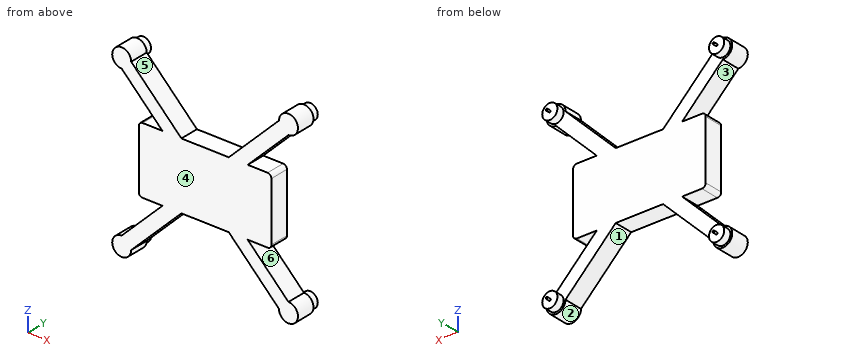
Autodesk Inventor part; units mm, degrees
ref_plane "YZ Plane" through (0, 0, 0) normal (1, 0, 0) x (0, 1, 0)
ref_plane "XZ Plane" through (0, 0, 0) normal (0, 1, 0) x (-1, 0, 0)
ref_plane "XY Plane" through (0, 0, 0) normal (0, 0, 1) x (1, 0, 0)
sketch "Sketch1" plane through (0, 0, 0) normal (0, 1, 0) x (-1, 0, 0)
  line L0 (49, 49) -> (-49, 49)
  line L1 (-49, 49) -> (-49, -49)
  line L2 (-49, -49) -> (49, -49)
  line L3 (49, -49) -> (49, 49)
  line L4 (49, 49) -> (-49, -49)
  line L5 (49, -49) -> (-49, 49)
  circle A0 centre (44, 44) radius 5
  line L6 (0, 0) -> (0, 5)
  line L7 (0, 0) -> (5, 0)
  line L8 (5, 0) -> (44, 39)
  line L9 (39, 44) -> (0, 5)
  circle A1 centre (-44, 44) radius 5
  line L10 (-44, 39) -> (-5, 0)
  line L11 (0, 5) -> (-39, 44)
  circle A2 centre (-44, -44) radius 5
  line L12 (-39, -44) -> (0, -5)
  line L13 (-5, 0) -> (-44, -39)
  circle A3 centre (44, -44) radius 5
  line L14 (44, -39) -> (5, 0)
  line L15 (0, -5) -> (39, -44)
  line L16 (-33, 17.5) -> (33, 17.5)
  line L17 (35, 15.5) -> (35, -15.5)
  line L18 (33, -17.5) -> (-33, -17.5)
  line L19 (-35, -15.5) -> (-35, 15.5)
  line L20 (-35, 17.5) -> (35, -17.5) construction
  line L21 (35, 17.5) -> (-35, -17.5) construction
  arc A4 (35, 15.5) -> (33, 17.5) centre (33, 15.5) ccw
  arc A5 (33, -17.5) -> (35, -15.5) centre (33, -15.5) ccw
  arc A6 (-35, -15.5) -> (-33, -17.5) centre (-33, -15.5) ccw
  arc A7 (-33, 17.5) -> (-35, 15.5) centre (-33, 15.5) ccw
  point P0 (12.5, 17.5)
  point P1 (-12.5, 17.5)
  point P2 (-22.5, 17.5)
  point P3 (-22.5, -17.5)
  point P4 (-12.5, -17.5)
  point P5 (12.5, -17.5)
  point P6 (22.5, -17.5)
  point P7 (22.5, 17.5)
  dimension "d0" = 98
  dimension "d1" = 98
  dimension "d2" = 10
  dimension "d3" = 49
  dimension "d4" = 49
  dimension "d7" = 360
  dimension "d10" = 70
  dimension "d11" = 35
  dimension "d12" = 2
  dimension "d13" = 2
  dimension "d14" = 2
  dimension "d15" = 2
extrude "Extrusion1" add sketch "Sketch1" along normal blind 10 contours A0 L4 | A0 L4 | A1 L5 | A0 L4 L16 L9 | A3 L5 | L8 L16 L4 A0 | L11 L16 L5 A1 | L5 A1 | L16 L4 L6 L9 | L9 L11 L16 | A3 L5 L18 L14 | A3 L5 | L16 A4 L17 A5 L18 L14 L8 | L8 L7 L4 L16 | L5 L16 L10 A1 | L11 L6 L5 L16 | A3 L15 L18 L5 | L18 L5 L7 L14 | L5 L18 L15 L12 L4 | L4 L18 L13 L10 L16 L5 | A2 L4 | A2 L4 | L18 L12 A2 L4 | L4 A2 L13 L18 | L10 L13 L18 A6 L19 A7 L16 | L18 L12 L15
sketch "Sketch2" plane through (0, 10, 0) normal (0, 1, 0) x (1, 0, 0)
  arc A0 (-44, -39) -> (-39, -44) centre (-44, -44) ccw
  circle A1 centre (-44, -44) radius 4
  arc A2 (-39, 44) -> (-44, 39) centre (-44, 44) ccw
  circle A3 centre (-44, 44) radius 4
  arc A4 (44, 39) -> (39, 44) centre (44, 44) ccw
  circle A5 centre (44, 44) radius 4
  arc A6 (39, -44) -> (44, -39) centre (44, -44) ccw
  circle A7 centre (44, -44) radius 4
  point P0 (0, 0)
  dimension "d18" = 8
  dimension "d19" = 8
  dimension "d20" = 8
  dimension "d21" = 8
extrude "Extrusion2" add sketch "Sketch2" along normal blind 4
sketch "Sketch3" plane through (-44, 14, 44) normal (0, 1, 0) x (1, 0, 0)
  circle A0 centre (0, 0) radius 0.5
  point P0 (44, 44)
  dimension "d24" = 1
sketch "Sketch4" plane through (-44, 14, -44) normal (0, 1, 0) x (1, 0, 0)
  circle A0 centre (0, 0) radius 4
  circle A1 centre (0, 0) radius 0.5
  point P0 (44, -44)
  dimension "d25" = 1
sketch "Sketch5" plane through (44, 14, -44) normal (0, 1, 0) x (1, 0, 0)
  circle A0 centre (0, 0) radius 4
  circle A1 centre (0, 0) radius 0.5
  point P0 (-44, -44)
  dimension "d26" = 1
sketch "Sketch6" plane through (44, 14, 44) normal (0, 1, 0) x (1, 0, 0)
  circle A0 centre (0, 0) radius 4
  circle A1 centre (0, 0) radius 0.5
  point P0 (-44, 44)
  dimension "d27" = 1
extrude "Extrusion3" add sketch "Sketch6" along normal blind 2 contours A1
extrude "Extrusion4" add sketch "Sketch3" along normal blind 2
extrude "Extrusion5" add sketch "Sketch4" along normal blind 2 contours A1
extrude "Extrusion6" add sketch "Sketch5" along normal blind 2 contours A1
properties part number "DroneBase"
Build history of the part. All positions in model axes, mm. Face numbers are marked on the shaded views. A direction names the side the tool comes from. Coordinates: 2 decimals unless noted, no trailing zeros. Order: outer loops, then holes, each group sorted by start corner. A loop starts at its lowest first (then second) coordinate and runs counter-clockwise, first axis right, second up. Notation, with made-up numbers: M 83,-36 L 102,-36 A12 ccw 102,-31 Z; hole C 17,-39 d9. An arc over 180 degrees is marked long. One line per question, with ' | ' between items. Start each with the question number.
1. Mould opens along X. For the marked faces 4, 5 and 6 say: +X half, -X half, draft (parallel to the pull), parting line (faces both ways), or undercut.
2. Cut at B-B (y = 5). Write the cut outline in (x, z), plus the area to 3 significant figures.
3. Flat gauge pins, fed straight in: P1, Ø8, axis at x = 30, y = 6, coming from the +Z side; P2, Ø3, axis at x = 5.5, y = 3, coming from the -Z side; P3, Ø5, axis at y = 3.5, z = 4.5, coming from the +X side; P4, Ø5, axis at y = 13, z = 13, coming from the +X side. Where does each tip first touch, or does it go through?
4. Cut at D-D (x = -9). Write the cut outline in (y, z), plus the area to 3 significant figures.
5. Cut at C-C (z = 9). Write the cut outline in (x, y), plus the area to 3 significant figures.
6. Wall check: line 1 along Z through (x, y) = (-25, 3); line 2 along Z through (x, y) = (31.5, 3.25); line 3 along Z through (x, y) = (44, 2). Give the ranges that are in metal, low to high. Write a range as [from, to].
7. Tool access for the marked faces 1, 2 and 3: list every direction of +Z, -Z, +X, -X, +Y, -Y with a clear straight run to the whole face (end or side of a thin tool).
8. Cut at A-A (z = -20). Write the cut outline in (x, y).
The answers:
1) face 4: draft | face 5: undercut | face 6: +X half
2) outline: M -44,-39 A5 ccw long -39,-44 L -12.5,-17.5 L 12.5,-17.5 L 39,-44 A5 ccw long 44,-39 L 22.5,-17.5 L 33,-17.5 A2 ccw 35,-15.5 L 35,15.5 A2 ccw 33,17.5 L 22.5,17.5 L 44,39 A5 ccw long 39,44 L 12.5,17.5 L -12.5,17.5 L -39,44 A5 ccw long -44,39 L -22.5,17.5 L -33,17.5 A2 ccw -35,15.5 L -35,-15.5 A2 ccw -33,-17.5 L -22.5,-17.5 Z | area: 3,690 mm2
3) P1: stops at z = 39 | P2: stops at z = -17.5 | P3: stops at x = 35 | P4: passes through
4) outline: M 0,-17.5 L 10,-17.5 L 10,17.5 L 0,17.5 Z | area: 350 mm2
5) outline: M -35,0 L 35,0 L 35,10 L -35,10 Z | area: 700 mm2
6) line 1: z = [-30, -20], [-17.5, 17.5], [20, 30] | line 2: z = [-36.5, -26.5], [-17.5, 17.5], [26.5, 36.5] | line 3: z = [-49, -39], [39, 49]
7) face 1: -Z, +Y, -Y | face 2: +Y, -Y | face 3: -X, +Y, -Y
8) outline: M -25,0 L -15,0 L -15,10 L -25,10 Z; M 15,0 L 25,0 L 25,10 L 15,10 Z
